Geometry: final body of the model. Coordinates: model frame, mm. Face numbers are marked on the shaded views. A direction names the side the tool comes from. Give positions to 0.01 mm unless a question says otherwise; leave off trailing zeros. Write each loop counter-clockwise with the first axis right and the second up, starting at its lowest first coordinate (ties: lowest second). Pieces come first, ordered by that corner, then holes. Notation, with made-up numbers: (-16, -40) -> (16, -40) arc R5 ccw to (16, -36) -> close; hole circle Ø9 at (-38, 34.5). An arc over 180 degrees is marked (long way). Answer as a JSON object with one key per item and string values.
from build123d import *

# Parameters (mm, degrees)
SKETCH1_R                = 14.15
SKETCH1_R_2              = 1.8
BOSS_EXTRUDE1_DEPTH      = 1.2
BOSS_EXTRUDE2_START      = -15
SKETCH3_R                = 15.35
SKETCH3_R_2              = 14.15
BOSS_EXTRUDE2_DEPTH      = 15
CUT_EXTRUDE2_DEPTH       = 8
BOSS_EXTRUDE3_REACH      = 43.566
BOSS_EXTRUDE3_END_RADIUS = 15.35
SKETCH6_W                = 15
SKETCH6_H                = 1.064778235
CIRPATTERN1_COUNT        = 2
CIRPATTERN1_ANGLE        = 305
SKETCH7_R                = 2.75
SKETCH7_R_2              = 1.75
BOSS_EXTRUDE4_DEPTH      = 4
FILLET1_R                = 4
SKETCH8_W                = 3.5
SKETCH8_H                = 15.633258876
CUT_EXTRUDE3_DEPTH       = 4
SKETCH4_R                = 1.5
CUT_EXTRUDE1_DEPTH       = 37


with BuildPart() as part:
    # Sketch1 → Boss-Extrude1 (new body)
    with BuildSketch(Plane.XY):
        Circle(SKETCH1_R)
        Circle(SKETCH1_R_2, mode=Mode.SUBTRACT)
    extrude(amount=BOSS_EXTRUDE1_DEPTH)

    # Sketch3 → Boss-Extrude2 (add)
    with BuildSketch(Plane.XY.offset(1.2).offset(BOSS_EXTRUDE2_START)):
        Circle(SKETCH3_R)
        Circle(SKETCH3_R_2, mode=Mode.SUBTRACT)
    extrude(amount=BOSS_EXTRUDE2_DEPTH)

    # Sketch5 → Cut-Extrude2 (cut)
    with BuildSketch(Plane(origin=(0, 0, -13.8), x_dir=(-1, 0, 0), z_dir=(0, 0, -1))):
        with BuildLine():
            Line((14.252659556, 5.699490817), (13.047619315, 5.47559405))
            ThreePointArc((13.047619315, 5.47559405), (13.871667407, 2.792730446), (14.15, 0))
            ThreePointArc((14.15, 0), (14.148415567, -0.21174737), (14.143662622, -0.423447319))
            Line((14.143662622, -0.423447319), (15.348702863, -0.199550552))
            ThreePointArc((15.348702863, -0.199550552), (15.349675712, -0.099777384), (15.35, 0))
            ThreePointArc((15.35, 0), (15.073168615, 2.902083373), (14.252659556, 5.699490817))
        make_face()
        with BuildLine():
            ThreePointArc((12.000869192, -7.496775216), (10.138626321, -9.870701916), (7.815412549, -11.79583938))
            Line((7.815412549, -11.79583938), (8.693613767, -12.650833161))
            ThreePointArc((8.693613767, -12.650833161), (10.998439154, -10.707793245), (12.87907041, -8.351768997))
            Line((12.87907041, -8.351768997), (12.000869192, -7.496775216))
        make_face()
    extrude(amount=-CUT_EXTRUDE2_DEPTH, mode=Mode.SUBTRACT)

    # Boss-Extrude3: up to this cylinder (the profile starts outside it)
    boss_extrude3_end = Plane(origin=(0, 0, -6.3), z_dir=(0, 0, 1)) * Cylinder(BOSS_EXTRUDE3_END_RADIUS, 118.832, mode=Mode.PRIVATE)
    # Sketch6 → Boss-Extrude3 (add, up to the surface)
    with BuildSketch(Plane(origin=(-12.463353061, -12.28473974, 0), x_dir=(0, 0, 1), z_dir=(-0.7121916034988102, -0.7019851279804962, 0)), mode=Mode.PRIVATE) as boss_extrude3_sk1:
        with Locations((-6.3, -3.782389118)):
            Rectangle(SKETCH6_W, SKETCH6_H)
    boss_extrude3_tool1 = extrude(boss_extrude3_sk1.sketch, amount=-BOSS_EXTRUDE3_REACH, mode=Mode.PRIVATE) - boss_extrude3_end
    # Sketch6 → Boss-Extrude3 (add, up to the surface)
    with BuildSketch(Plane(origin=(-12.463353061, -12.28473974, 0), x_dir=(0, 0, 1), z_dir=(-0.7121916034988102, -0.7019851279804962, 0)), mode=Mode.PRIVATE) as boss_extrude3_sk2:
        with Locations((-6.3, 3.782389118)):
            Rectangle(SKETCH6_W, SKETCH6_H)
    boss_extrude3_tool2 = extrude(boss_extrude3_sk2.sketch, amount=-BOSS_EXTRUDE3_REACH, mode=Mode.PRIVATE) - boss_extrude3_end
    boss_extrude3 = boss_extrude3_tool1.solids().sort_by_distance((-9.808172, -14.978526, -6.3))[0] + boss_extrude3_tool2.solids().sort_by_distance((-15.118534, -9.590954, -6.3))[0]
    add(boss_extrude3)

    # CirPattern1: Boss-Extrude3 ×2 about axis
    cirpattern1_axis = Axis((0, 0, 0), (0, 0, 1))
    for i in range(1, CIRPATTERN1_COUNT):
        add(boss_extrude3.rotate(cirpattern1_axis, i * CIRPATTERN1_ANGLE / (CIRPATTERN1_COUNT - 1)))

    # Sketch7 → Boss-Extrude4 (add)
    with BuildSketch(Plane(origin=(0, 0, 0), x_dir=(-1, 0, 0), z_dir=(0, 0, -1))):
        with Locations(Location((0, 0, 0), (0, 0, 180))):
            Circle(SKETCH7_R)
        Circle(SKETCH7_R_2, mode=Mode.SUBTRACT)
    extrude(amount=BOSS_EXTRUDE4_DEPTH)

    # Fillet1
    fillet1_edges = [part.edges().sort_by_distance(p)[0] for p in [
        (-2.75, 0, 0),
    ]]
    fillet(fillet1_edges, radius=FILLET1_R - 0.0001)  # a hair under: the kernel refuses the full size

    # Sketch8 → Cut-Extrude3 (cut)
    with BuildSketch(Plane(origin=(0, 0, -4), x_dir=(-1, 0, 0), z_dir=(0, 0, -1))):
        Rectangle(SKETCH8_W, SKETCH8_H)
    extrude(amount=-CUT_EXTRUDE3_DEPTH, mode=Mode.SUBTRACT)

    # Sketch4 → Cut-Extrude1 (cut)
    with BuildSketch(Plane(origin=(-17.515032447, -2.63115554, 0), x_dir=(0.293814927975495, -0.9558623269586236, 0), z_dir=(0.9558623269586236, 0.293814927975495, 0))):
        with Locations((2.63115554, 1.8)):
            Circle(SKETCH4_R)
    extrude(amount=CUT_EXTRUDE1_DEPTH, mode=Mode.SUBTRACT)


solid = part.part
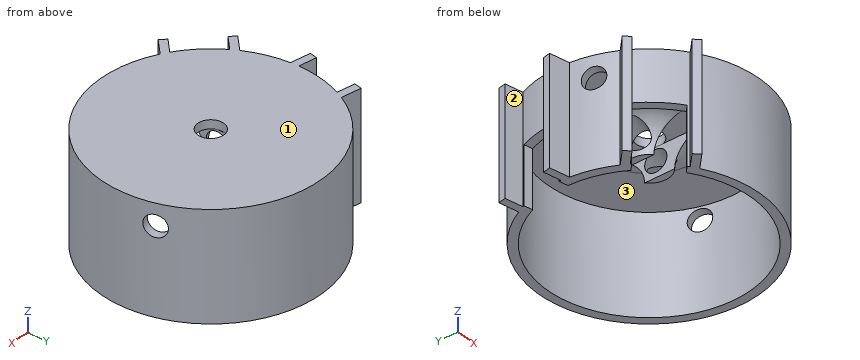
Q1. Cut plane D-D (y = 8). Return the cut outline in (x, z), and give its area (3 significant figures).
Values:
{"outline": "(-13.1, -13.8) -> (-11.67, -13.8) -> (-11.67, 0) -> (11.67, 0) -> (11.67, -13.8) -> (13.1, -13.8) -> (13.1, 1.2) -> (-13.1, 1.2) -> close", "area": "70.9 mm²"}
Q2. Cut plane A-A (z = -4.75). Return the cut outline in (x, y).
Values:
{"outline": "(-17.99, -1.08) -> (-15.27, -1.58) arc R15.35 ccw to (-13.52, -7.27) -> (-15.49, -9.21) -> (-14.74, -9.97) -> (-12.97, -8.22) arc R15.35 ccw to (-8.4, -12.85) -> (-10.18, -14.6) -> (-9.43, -15.36) -> (-7.46, -13.41) arc R15.35 ccw (long way) to (-13.71, 6.91) -> (-16.43, 7.41) -> (-16.62, 6.36) -> (-14.17, 5.91) arc R15.35 ccw to (-15.34, -0.48) -> (-17.8, -0.03) -> close; hole circle Ø28.3 at (0, 0)"}
Q3. First-contact query: P1, Ø2.5, axis at x = -9.5, y = -11, coming from the -Z side; P2, Ø5, axis at x = -8.5, z = -8.5, coming from the -Y side; P3, Ø1.2, axis at y = -1, z = -2.5, coming from the +X side. Flat tips, straight axial feed; report the tip coordinate or a pass-through.
Values:
{"P1": "z = -5.8", "P2": "y = -15.36", "P3": "x = 15.34"}
Q4. Material intervals for L1, parallel to Y at x = -0.5, z = -10.25; L2, parallel to X at y = -9, z = -4; L3, parallel to Y at x = -9, z = -3.75, sorted ascending. Write a range as from..to.
Values:
{"L1": "-15.34..-14.14, 14.14..15.34", "L2": "-15.28..-13.76, -12.43..-10.92, 10.92..12.43", "L3": "-14.93..-13.43, -12.43..-10.92, 10.92..12.43"}
Q5. Cut plane B-B (x = 0). Return the cut outline in (y, z).
Values:
{"outline": "(-15.35, -13.8) -> (-14.15, -13.8) -> (-14.15, 0) -> (-1.8, 0) -> (-1.8, 1.2) -> (-15.35, 1.2) -> close; (1.8, 0) -> (14.15, 0) -> (14.15, -13.8) -> (15.35, -13.8) -> (15.35, 1.2) -> (1.8, 1.2) -> close"}
Q6. Cut plane C-C (z = -7.75). Return the cut outline in (x, y).
Values:
{"outline": "(-17.99, -1.08) -> (-15.27, -1.58) arc R15.35 ccw to (-13.52, -7.27) -> (-15.49, -9.21) -> (-14.74, -9.97) -> (-12.97, -8.22) arc R15.35 ccw to (-12.88, -8.35) -> (-12, -7.5) arc R14.15 cw to (-14.14, -0.42) -> (-15.35, -0.2) arc R15.35 ccw to (-15.34, -0.48) -> (-17.8, -0.03) -> close; (-16.62, 6.36) -> (-14.17, 5.91) arc R15.35 ccw to (-14.25, 5.7) -> (-13.05, 5.48) arc R14.15 cw (long way) to (-7.82, -11.8) -> (-8.69, -12.65) arc R15.35 ccw to (-8.4, -12.85) -> (-10.18, -14.6) -> (-9.43, -15.36) -> (-7.46, -13.41) arc R15.35 ccw (long way) to (-13.71, 6.91) -> (-16.43, 7.41) -> close"}
Q7. Set-up query: the marked faces 1, 2 and 3. Return all of +Z, -Z, +X, -X, +Y, -Y with unobstructed straight access to the full face (end or side cutting, diameter ignored); none if empty.
Values:
{"face 1": "+Z, +X, -X, +Y, -Y", "face 2": "+Z, -Z, -X", "face 3": "-Z"}
